Autodesk Inventor part; units mm, degrees
ref_plane "YZ Plane" through (0, 0, 0) normal (1, 0, 0) x (0, 1, 0)
ref_plane "XZ Plane" through (0, 0, 0) normal (0, 1, 0) x (-1, 0, 0)
ref_plane "XY Plane" through (0, 0, 0) normal (0, 0, 1) x (1, 0, 0)
sketch "Main Sketch" plane through (0, 0, 0) normal (0, 1, 0) x (-1, 0, 0)
  line L0 (-44.375, -9.3176) -> (-44.375, 9.3176)
  line L1 (-44.375, 9.3176) -> (47.625, -10) construction
  line L2 (47.625, 10) -> (-44.375, -9.3176) construction
  circle A0 centre (47.625, 0) radius 7
  arc A1 (47.625, -10) -> (47.625, 10) centre (47.625, 0) ccw
  line L3 (-27.875, 17.5) -> (-44.375, 17.5)
  line L4 (-44.375, 17.5) -> (-44.375, -17.5)
  line L5 (-44.375, -17.5) -> (-27.875, -17.5)
  line L6 (-27.875, 17.5) -> (-44.375, -17.5) construction
  line L7 (-44.375, 17.5) -> (-27.875, -17.5) construction
  line L8 (47.625, -10) -> (-27.875, -10)
  line L9 (-27.875, -17.5) -> (-27.875, -10)
  line L10 (-27.875, 10) -> (-27.875, 17.5)
  line L11 (-27.875, 10) -> (47.625, 10)
  point P0 (0, 0)
  point P1 (-36.125, 0)
  dimension "d3" = 14
  dimension "d4" = 92
  dimension "d13" = 16.5
  dimension "d14" = 35
  dimension "d15" = 0
  dimension "d18" = 20
extrude "Main Extrusion" add sketch "Main Sketch" along normal blind 4
sketch "Screw Holes Sketch" plane through (0, 4, 0) normal (0, 1, 0) x (1, 0, 0)
  circle A0 centre (33.125, -8.75) radius 2
  line L0 (44.375, 17.5) -> (27.875, 17.5)
  line L1 (27.875, -17.5) -> (44.375, -17.5)
  line L2 (22.2664, 0) -> (52.7891, 0)
  line L3 (38.375, -27.0398) -> (38.375, 30.2346) construction
  line L4 (44.375, -17.5) -> (44.375, 17.5)
  line L5 (27.875, -10) -> (27.875, -17.5)
  circle A1 centre (33.125, 8.75) radius 2
  line L6 (38.375, 27.0398) -> (38.375, -30.2346) construction
  point P0 (0, 0)
  dimension "d21" = 4
  dimension "d22" = 35
  dimension "d23" = 6
  dimension "d24" = 5.25
  dimension "d25" = 5.25
  dimension "d26" = 10.5
  dimension "d27" = 8.75
  dimension "d28" = 17.5
extrude "Screw Holes Cut" cut sketch "Screw Holes Sketch" against normal through all
fillet "Smoooooooooooooooooth" radius 6 2 edges at (27.875, 2, -17.5) (27.875, 2, 17.5)
sketch "Side Axel Hole Sketch" plane through (-47.625, 0, 10) normal (0, 0, 1) x (1, 0, 0)
  line L0 (75.5, 4) -> (75.5, 0)
  line L1 (0, 0) -> (0, 4)
  line L2 (44.25, -12.0383) -> (44.25, 22.7681) construction
  line L3 (75.5, 0) -> (0, 0)
  line L4 (0, 4) -> (75.5, 4)
  circle A0 centre (44.25, 4) radius 1.5
  point P0 (47.625, 0)
  dimension "d32" = 75.5
  dimension "d33" = 44.25
  dimension "d34" = 31.25
  dimension "d35" = 4
  dimension "d41" = 3
extrude "Side Axel Hole Cut" cut sketch "Side Axel Hole Sketch" against normal blind 20 contours A0 L4 | L4 A0
sketch "Side Hole Extension Sketch" plane through (-47.625, 0, 10) normal (0, 0, 1) x (1, 0, 0)
  arc A0 (42.75, 4) -> (45.75, 4) centre (44.25, 4) ccw
  circle A1 centre (44.25, 4) radius 3
  circle A2 centre (44.25, 4) radius 1.5
  point P0 (47.625, 0)
  dimension "d44" = 6
extrude "Side Hole Extrusion" add sketch "Side Hole Extension Sketch" against normal blind 20
sketch "Body Holes Sketch" plane through (0, 4, 0) normal (0, 1, 0) x (1, 0, 0)
  line L0 (-37.625, 8) -> (-8.375, 8)
  line L1 (-8.375, 8) -> (-8.375, 4)
  line L2 (-8.375, 4) -> (-37.625, 4)
  line L3 (-37.625, 4) -> (-37.625, 8)
  line L4 (-6.375, -10) -> (-6.375, 10)
  circle A0 centre (-47.625, 0) radius 7
  line L5 (-47.625, 7) -> (-47.625, -13.5384) construction
  line L6 (-6.375, 10) -> (-47.625, 10)
  line L7 (-47.625, 1) -> (-47.625, -19.5384) construction
  line L8 (-37.625, 2) -> (-8.375, 2)
  line L9 (-8.375, 2) -> (-8.375, -2)
  line L10 (-8.375, -2) -> (-37.625, -2)
  line L11 (-37.625, -2) -> (-37.625, 2)
  line L12 (-47.625, -5) -> (-47.625, -25.5384) construction
  line L13 (-37.625, -4) -> (-8.375, -4)
  line L14 (-8.375, -4) -> (-8.375, -8)
  line L15 (-8.375, -8) -> (-37.625, -8)
  line L16 (-37.625, -8) -> (-37.625, -4)
  line L17 (1.625, 8) -> (26.625, 8)
  line L18 (26.625, 8) -> (26.625, 4)
  line L19 (26.625, 4) -> (1.625, 4)
  line L20 (1.625, 4) -> (1.625, 8)
  line L21 (-0.375, 10) -> (-0.375, -10)
  line L22 (27.875, 10) -> (-0.375, 10)
  line L23 (1.625, -2) -> (1.625, 2)
  line L24 (26.625, -2) -> (1.625, -2)
  line L25 (26.625, 2) -> (26.625, -2)
  line L26 (1.625, 2) -> (26.625, 2)
  line L27 (1.625, -8) -> (1.625, -4)
  line L28 (26.625, -8) -> (1.625, -8)
  line L29 (26.625, -4) -> (26.625, -8)
  line L30 (1.625, -4) -> (26.625, -4)
  point P0 (0, 0)
  dimension "d77" = 4
  dimension "d78" = 2
  dimension "d79" = 10
  dimension "d80" = 2
  dimension "d83" = 6
  dimension "d88" = 2
  dimension "d89" = 2
  dimension "d90" = 4
  dimension "d91" = 25
  dimension "d94" = 6
extrude "Swiss-ified" cut sketch "Body Holes Sketch" against normal through all contours L0 L1 L2 L3 | L8 L9 L10 L11 | L13 L14 L15 L16 | L17 L18 L19 L20 | L23 L26 L25 L24 | L27 L30 L29 L28
properties part number "Side V4"
For this review, take the finished solid that the model builds, in its own axes (mm). A direction names the side the tool comes from. Coordinates: 2 decimals unless noted, no trailing zeros. Order: outer loops, then holes, each group sorted by start corner. A loop starts at its lowest first (then second) coordinate and runs counter-clockwise, first axis right, second up. Notation, with made-up numbers: (74, 5.5) -> (97, 5.5) arc R33 cw to (97, 34.5) -> close; hole circle Ø5 at (28.25, -31). An arc over 180 degrees is marked (long way). Return JSON: item names as keys, results as strings.
1. Machinability: for faces 5 (the flat face through (-10, 2, -10)), 6 (the flat face through (-31.6, 4, 2.4)), 7 (the flat face through (-23, 2, 4)), which of the approach directions +Z, -Z, +X, -X, +Y, -Y give a long, thin tool a straight path to every point of the face, cutting with its end or side? Answer none if there is none.
Answer block:
{"face 5": "-Z, -X, +Y, -Y", "face 6": "+Z, -Z, -X, +Y", "face 7": "+Y, -Y"}
2. We need section B-B on x = 9.5. Write out the cut boundary in (y, z).
Answer block:
{"outline": "(0, -10) -> (4, -10) -> (4, -8) -> (0, -8) -> close; (0, -4) -> (4, -4) -> (4, -2) -> (0, -2) -> close; (0, 2) -> (4, 2) -> (4, 4) -> (0, 4) -> close; (0, 8) -> (4, 8) -> (4, 10) -> (0, 10) -> close"}
3. We need section C-C on x = -50. Write out the cut boundary in (y, z), and give its area (3 significant figures).
Answer block:
{"outline": "(0, -9.71) -> (4, -9.71) -> (4, -6.58) -> (0, -6.58) -> close; (0, 6.58) -> (4, 6.58) -> (4, 9.71) -> (0, 9.71) -> close", "area": "25.0 mm²"}
4. We need section A-A on z = 0. Write out the cut boundary in (x, y) (3 decimals).
Answer block:
{"outline": "(-57.625, 0) -> (-54.625, 0) -> (-54.625, 4) -> (-57.625, 4) -> close; (-40.625, 0) -> (-37.625, 0) -> (-37.625, 4) -> (-40.625, 4) -> close; (-8.375, 0) -> (1.625, 0) -> (1.625, 4) -> (-0.375, 4) arc R3 ccw to (-6.375, 4) -> (-8.375, 4) -> close; (26.625, 0) -> (44.375, 0) -> (44.375, 4) -> (26.625, 4) -> close; hole circle Ø3 at (-3.375, 4)"}
5. For line 1 (Z direction, x = -27.5, y = 1); line 2 (Y direction, x = 11, z = -2.5); line 3 (Z direction, x = -45, y = 3.5), list the stretches that pass through material, from the lowest coordinate up. Write a range as from..to.
Answer block:
{"line 1": "-10..-8, -4..-2, 2..4, 8..10", "line 2": "0..4", "line 3": "-10..-6.49, 6.49..10"}
6. We need section D-D on y = 1. State how many separate pieces and enclosed holes the cut face has, and give its area (3 significant figures).
Answer block:
{"separate pieces": "1", "enclosed holes": "9", "area": "1,400 mm²"}
7. The part is to be moulded in two halves that separate along X. For faces 1 (the cylindrical face through (-54.302, 1.972, -2.103)), 2 (the flat face through (26.625, 2, 0)), 3 (the flat face through (39, 2, 17.5)), 4 (the cylindrical face through (-3.3, 7, 0.1)), say which applies: +X half, -X half, draft (parallel to the pull), parting line (faces both ways), or undercut.
Answer block:
{"face 1": "undercut", "face 2": "undercut", "face 3": "draft", "face 4": "parting line"}
8. For pin 1 Ø12 at (x, z) = (-17, -12) entering from -Y; pin 2 Ø2 at (y, z) = (3, 2) entering from -X; pin 3 Ø3 at (x, y) = (-15, 5) entering from -Z; pin 4 Ø0.8 at (y, z) = (2.5, -11) entering from -X (3 decimals), all flat-tipped, find the tip position at first contact; note any pin that passes through.
Answer block:
{"pin 1": "y = 0", "pin 2": "x = -57.57", "pin 3": "z = -10", "pin 4": "x = 27.875"}
